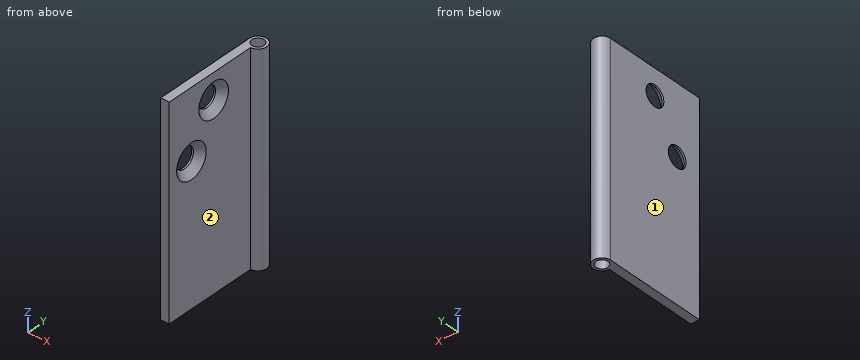
from build123d import *

# Parameters (mm, degrees)
SKETCH_1_W                  = 5
SKETCH_1_H                  = 60
EXTRUDE_2_DEPTH             = 60
SKETCH_2_R                  = 5
SKETCH_3_R                  = 3.5
CUT_EXTRUDE_1_DEPTH         = 137.839321834
HOLE_WIZARD_M101_AT_2_COUNT = 2
HOLE_WIZARD_M101_AT_2_PITCH = 29.154759474


with BuildPart() as part:
    # Эскиз1 → Вытянуть-Тонкостенный2 (new, symmetric)
    with BuildSketch(Plane.XY):
        with Locations((2.5, 30)):
            Rectangle(SKETCH_1_W, SKETCH_1_H)
    extrude(amount=EXTRUDE_2_DEPTH, both=True)

    # По траектории1: sweep along a curve in space
    with BuildLine() as sweep_1_path:
        Line((0, 60, 60), (0, 60, -60))
    # Эскиз2 → По траектории1 (sweep)
    with BuildSketch(Plane.XY.offset(60)):
        with Locations((5, 60)):
            Circle(SKETCH_2_R)
    sweep(path=sweep_1_path.line)

    # Эскиз3 → Вырез-Вытянуть1 (cut, through all)
    with BuildSketch(Plane.XY.offset(60)):
        with Locations((5, 60)):
            Circle(SKETCH_3_R)
    extrude(amount=-CUT_EXTRUDE_1_DEPTH, mode=Mode.SUBTRACT)

    # Эскиз8 → Зенковка для  винта с плоской головкой M101 (revolve, cut)
    with BuildSketch(Plane(origin=(5, 30, 45), x_dir=(0, 0, -1), z_dir=(0, 1, 0))):
        Polygon((0, 0), (0, 5), (6, 5), (6, 4), (10, 0), align=None)
    hole_wizard_m101 = revolve(axis=Axis((11.35, 30, 45), (-1, 0, 0)), mode=Mode.SUBTRACT)

    # Зенковка для  винта с плоской головкой M101 at 2: Зенковка для  винта с плоской головкой M101 ×2
    with Locations(*[Vector(0, -0.5144957554275265, -0.8574929257125442) * (i * HOLE_WIZARD_M101_AT_2_PITCH) for i in range(1, HOLE_WIZARD_M101_AT_2_COUNT)]):
        add(hole_wizard_m101, mode=Mode.SUBTRACT)


solid = part.part
Verification items for the finished model (mm, model axes). Face numbers are marked on the shaded views. A direction names the side the tool comes from. Give positions to 0.01 mm unless a question says otherwise; leave off trailing zeros. Order: outer loops, then holes, each group sorted by start corner. A loop starts at its lowest first (then second) coordinate and runs counter-clockwise, first axis right, second up. Notation, with made-up numbers: M 79.5,18 L 95.5,18 A16 cw 95.5,29 Z; hole C -33.5,59 d1. An arc over 180 degrees is marked long. Use one line per item in the form item = value. Start each with the question number.
Q1. Go/stop test with flat-tipped pins: pin 1 Ø1.5 at (x, z) = (9, -35) entering from -Y; pin 2 Ø5.5 at (x, y) = (5, 60) entering from -Z; pin 3 Ø2 at (x, z) = (6.5, 11) entering from -Y; pin 4 Ø14 at (y, z) = (30, 45) entering from +X. Record where each tip stops, or that it passes through.
Q2. Section check C-C (x = 2.75). Enter the section's corners in (y, z).
Q3. Section check A-A (z = 45). Enter the section's corners in (x, y).
Q4. Section check B-B (y = 30). Enter the section's corners in (x, z), then the cut area to 3 significant figures.
Q5. Access from +Z, -Z, +X, -X, +Y, -Y to the whole of each face (thin tool, end or side, straight path). Record for the marked faces 1 and 2.
Q6. Scan lines: line 1 along Z through (x, y) = (0.6, 30); line 2 along Y through (x, z) = (2, 20); line 3 along X through (y, z) = (49, -12.5). Record each from-to range of solid material in increasing order. Write a range as [from, to].
Q7. Section check D-D (z = -15.5). Enter the section's corners in (x, y), then the cut area to 3 significant figures.
Evaluation:
q1.pin_1 = 56.2
q1.pin_2 = through
q1.pin_3 = 55.03
q1.pin_4 = 2
q2.outline = M 0,-60 L 57.32,-60 L 57.32,60 L 0,60 Z; M 62.68,-60 L 64.47,-60 L 64.47,60 L 62.68,60 Z; hole C 15,20 d15.5; hole C 30,45 d15.5
q3.outline = M 0,0 L 5,0 L 5,20 L 1,24 L 0,24 Z; M 0,36 L 1,36 L 5,40 L 5,55 A5 ccw long 0,60 Z; hole C 5,60 d7
q4.outline = M 0,-60 L 5,-60 L 5,35 L 1,39 L 0,39 Z; M 0,51 L 1,51 L 5,55 L 5,60 L 0,60 Z
q4.area = 524 mm2
q5.face_1 = +Z, -Z, -X, +Y, -Y
q5.face_2 = +Z, -Z, +X, -Y
q6.line_1 = [-60, 39], [51, 60]
q6.line_2 = [0, 8], [22, 58.2], [61.8, 64]
q6.line_3 = [0, 5]
q7.outline = M 0,0 L 5,0 L 5,55 A5 ccw long 0,60 Z; hole C 5,60 d7
q7.area = 320 mm2
